Geometry: final body of the model. Coordinates: model frame, mm. A direction names the side the tool comes from. Coordinates: 2 decimals unless noted, no trailing zeros. Loops run counter-clockwise (first coordinate to the right, second up) from the corner with the lowest first, then second, coordinate; pieces in that order, holes last. Notation, with made-up numbers: (78, 53) -> (102, 53) arc R14 cw to (102, 79) -> close; hole circle Ø3 at (23.5, 53). An arc over 180 degrees is marked (long way). One line per item, written item: value. Start each with the question number.
Item 1: Section query A-A on x = 2. Return loops of the section in (y, z).
Item 2: Section query C-C on x = -80.5. Return loops of the section in (y, z).
Item 3: Section query B-B on y = 1.35. Return loops of the section in (x, z), then the cut area to 3 significant figures.
Item 4: Set-up query: faces 5 (the flat face through (-80, 1, 0)), 6 (the cylindrical face through (-4.89, 0.99, -5)). Return all of +Z, -Z, +X, -X, +Y, -Y with unobstructed straight access to the full face (end or side cutting, diameter ignored); none if empty.
Item 5: Mould query, pull axis Z, two halves, no side actions, for faces 1 (the cylindrical face through (-71.954, 0.986, -2.055)), 2 (the cylindrical face through (3.233, 0.986, 1.341)), 3 (the flat face through (-36, 0, -10)), 4 (the flat face through (-26.87, 0.99, 4.93)). Classes: +Z half, -Z half, draft (parallel to the pull), parting line (faces both ways), or undercut.
Item 6: Section query D-D on z = -15. Return loops of the section in (x, y).
Item 7: Contact query for a flat-ended pin moving along its axis: pin 1 Ø1 at (y, z) = (1.5, -7.5) entering from +X. Output: stop coordinate, or through.
Item 8: Ray query, probe 1 along X at (y, z) = (1.35, -2); probe 2 along Z at (x, y) = (0, 0.75); probe 3 along X at (y, z) = (0.95, -7.5). Return the intervals inside material, ascending. Write a range as from..to.
from build123d import *

# Parameters (mm, degrees)
SKETCH1_R           = 3.5
SKETCH1_R_2         = 1.25
SKETCH1_R_3         = 1.75
BOSS_EXTRUDE1_DEPTH = 2
FILLET_1_R          = 1


with BuildPart() as part:
    # Sketch1 → Boss-Extrude1 (new body)
    with BuildSketch(Plane(origin=(0, 0, 0), x_dir=(1, 0, 0), z_dir=(0, 1, 0))):
        with BuildLine():
            Line((-13.426718388, 22.622894631), (-86.83738777, 22.622894631))
            Line((-86.83738777, 22.622894631), (-108, 0))
            Line((-108, 0), (-53, 0))
            Line((-53, 0), (0, -10))
            ThreePointArc((0, -10), (7.071067812, -7.071067812), (10, 0))
            ThreePointArc((10, 0), (2.856758636, 16.043947959), (-13.426718388, 22.622894631))
        make_face()
        Circle(SKETCH1_R, mode=Mode.SUBTRACT)
        with Locations((-92.705183178, 2)):
            Circle(SKETCH1_R_2, mode=Mode.SUBTRACT)
        with Locations((-70.705183178, 2)):
            Circle(SKETCH1_R_2, mode=Mode.SUBTRACT)
        with Locations((-3.5, 6.062177826)):
            Circle(SKETCH1_R_3, mode=Mode.SUBTRACT)
        with Locations((7, 0)):
            Circle(SKETCH1_R_3, mode=Mode.SUBTRACT)
        with Locations((-3.5, -6.062177826)):
            Circle(SKETCH1_R_3, mode=Mode.SUBTRACT)
    extrude(amount=BOSS_EXTRUDE1_DEPTH)

    # Скругление1
    fillet_1_edges = [part.edges().sort_by_distance(p)[0] for p in [
        (-108, 1, 0),
    ]]
    fillet(fillet_1_edges, radius=FILLET_1_R)


solid = part.part
Reply:
1. outline: (0, -16.83) -> (2, -16.83) -> (2, -2.87) -> (0, -2.87) -> close; (0, 2.87) -> (2, 2.87) -> (2, 9.8) -> (0, 9.8) -> close
2. outline: (0, -22.62) -> (2, -22.62) -> (2, 0) -> (0, 0) -> close
3. outline: (-106.43, -1.68) -> (-86.84, -22.62) -> (-13.43, -22.62) arc R23.44 ccw to (10, 0) arc R10 ccw to (0, 10) -> (-53, 0) -> (-105.7, 0) arc R1 ccw to start; hole circle Ø2.5 at (-92.71, -2); hole circle Ø2.5 at (-70.71, -2); hole circle Ø3.5 at (-3.5, -6.06); hole circle Ø3.5 at (-3.5, 6.06); hole circle Ø7 at (0, 0); hole circle Ø3.5 at (7, 0)
3. area: 2,580 mm²
4. face 5: +Z, -X, +Y, -Y
4. face 6: +Y, -Y
5. face 1: undercut
5. face 2: undercut
5. face 3: draft
5. face 4: +Z half
6. outline: (-93.97, 0) -> (3.87, 0) -> (3.87, 2) -> (-93.97, 2) -> close
7. pin 1: stops at x = 8.67
8. probe 1: x = -106.13..-93.96, -91.46..-71.96, -69.46..-2.87, 2.87..9.84
8. probe 2: z = -18.4..-3.5, 3.5..10
8. probe 3: x = -100.98..-4.5, -2.5..8.49
